from build123d import *

# Parameters (mm, degrees)
F0_R     = 2.5
F0_R_2   = 11
F1_DEPTH = 2
F2_R     = 1.99999


# Not quite as in the source:
# - a fillet or chamfer is up to 0.001 mm smaller than in the source, because OpenCascade refuses the exact size


with BuildPart() as f1:
    # F0 (on Top) → F1 (new body, symmetric)
    with BuildSketch(Plane.XY):
        with BuildLine():
            ThreePointArc((22.0269415402, 27.1995192308), (0, 21.25), (-22.0269415402, 27.1995192308))
            ThreePointArc((-22.0269415402, 27.1995192308), (-30.3108891325, 17.5), (-34.5689453947, 5.4761313261))
            ThreePointArc((-34.5689453947, 5.4761313261), (-18.4030398304, -10.625), (-12.5420038545, -32.6756505569))
            ThreePointArc((-12.5420038545, -32.6756505569), (0, -35), (12.5420038545, -32.6756505569))
            ThreePointArc((12.5420038545, -32.6756505569), (18.4030398304, -10.625), (34.5689453947, 5.4761313261))
            ThreePointArc((34.5689453947, 5.4761313261), (30.3108891325, 17.5), (22.0269415402, 27.1995192308))
        make_face()
        with Locations((-6.4819163414, -28.1422128626)):
            Circle(F0_R, mode=Mode.SUBTRACT)
        with Locations((-8.6058037086, -17.4647100248)):
            Circle(F0_R, mode=Mode.SUBTRACT)
        with Locations((-12.9903810568, -7.5)):
            Circle(F0_R, mode=Mode.SUBTRACT)
        with Locations((6.4819163414, -28.1422128626)):
            Circle(F0_R, mode=Mode.SUBTRACT)
        with Locations((8.6058037086, -17.4647100248)):
            Circle(F0_R, mode=Mode.SUBTRACT)
        with Locations((12.9903810568, -7.5)):
            Circle(F0_R, mode=Mode.SUBTRACT)
        with Locations((-19.4277844055, 1.2795103808)):
            Circle(F0_R, mode=Mode.SUBTRACT)
        with Locations((-27.6128294284, 8.4576022144)):
            Circle(F0_R, mode=Mode.SUBTRACT)
        with Locations((-21.130913087, 19.6846106482)):
            Circle(F0_R, mode=Mode.SUBTRACT)
        with Locations((-10.8219806969, 16.185199644)):
            Circle(F0_R, mode=Mode.SUBTRACT)
        Circle(F0_R_2, mode=Mode.SUBTRACT)
        with Locations((19.4277844055, 1.2795103808)):
            Circle(F0_R, mode=Mode.SUBTRACT)
        with Locations((27.6128294284, 8.4576022144)):
            Circle(F0_R, mode=Mode.SUBTRACT)
        with Locations((0, 15)):
            Circle(F0_R, mode=Mode.SUBTRACT)
        with Locations((10.8219806969, 16.185199644)):
            Circle(F0_R, mode=Mode.SUBTRACT)
        with Locations((21.130913087, 19.6846106482)):
            Circle(F0_R, mode=Mode.SUBTRACT)
    extrude(amount=F1_DEPTH, both=True)

    # F2 (radius 2 in the source; OpenCascade refuses exactly that, so slightly less here)
    f2_edges = [f1.edges().sort_by_distance(p)[0] for p in [
        (0, -35, 2),
        (-18.40304, -10.625, 2),
        (30.310889, 17.5, 2),
        (-18.40304, -10.625, -2),
        (0, 21.25, -2),
        (0, 21.25, 2),
        (-30.310889, 17.5, -2),
        (-30.310889, 17.5, 2),
        (30.310889, 17.5, -2),
        (18.40304, -10.625, 2),
        (18.40304, -10.625, -2),
        (0, -35, -2),
    ]]
    fillet(f2_edges, radius=F2_R)


solid = f1.part
Work out the finished part from the listing and answer in its coordinate system (mm). Round coordinates to 2 decimals unless told otherwise and drop trailing zeros.
1) A cutting plane is placed at A-A (x = 0). Give the number of separate pieces and of enclosed holes in the cut face, plus the area to 3 significant figures.
2) The mould has two halves that part along Y. Classify faces 1 (the cylindrical face through (-4.097, -27.391, -0.028)), 2 (the flat face through (5, -10, 2)): pulls with the +Y half, pulls with the -Y half, needs draft (parallel to the pull), parting line crosses it, or undercut.
3) Straight lines are drawn through the part: line 1 (X direction, y = 2, z = 1.4); line 2 (X direction, y = -28, z = 0.25); line 3 (X direction, y = 16, z = -1.3). For each, find the intervals that lie inside material, in ascending order.
4) Given pin 1 Ø6.5 at (x, y) = (0, 15) entering from -Z; pin 2 Ø3 at (x, y) = (-8.61, -17.46) entering from +Z; pin 3 Ø1.5 at (x, y) = (26.5, 0) entering from +Z, each flat-ended and moving along its own axis, determine where each tip first touches the part or whether it passes through.
Completed:
1. separate pieces: 3
1. enclosed holes: 0
1. area: 114 mm2
2. face 1: undercut
2. face 2: needs draft
3. line 1: x = -28.47 to -21.82, -17.03 to -10.82, 10.82 to 17.03, 21.82 to 28.47
3. line 2: x = -12.76 to -8.98, -3.99 to 3.99, 8.98 to 12.76
3. line 3: x = -30.59 to -13.32, -8.33 to -2.29, 2.29 to 8.33, 13.32 to 30.59
4. pin 1: stops at z = -2
4. pin 2: passes through
4. pin 3: stops at z = 1.78
